CAD build for the part. Positions are in the model's coordinates, mm. A direction names the side the tool comes from. Give positions to 0.01 mm unless a question says otherwise; leave off trailing zeros. Write each loop counter-clockwise with the first axis right and the second up, starting at its lowest first coordinate (ties: lowest second). Pieces come first, ordered by that corner, then holes. Notation, with made-up numbers: (42.25, 40) - (63.25, 40) arc R21 cw to (63.25, 60) - close; hole circle Ø5 at (60.25, -23). An arc over 180 degrees is marked (long way). Answer as a JSON object with one key per item and string values.
from build123d import *

# Parameters (mm, degrees)
SKETCH1_R           = 0.19
SKETCH1_R_2         = 0.815
BOSS_EXTRUDE1_DEPTH = 1
SKETCH2_R           = 0.375
CUT_EXTRUDE1_DEPTH  = 0.75
SKETCH3_W           = 1.01
SKETCH3_H           = 1.01
CUT_EXTRUDE2_DEPTH  = 15
SKETCH4_R           = 0.125
CUT_EXTRUDE3_DEPTH  = 1.01
CHAMFER1_SIZE       = 0.05


with BuildPart() as part:
    # Sketch1 → Boss-Extrude1 (new body, symmetric)
    with BuildSketch(Plane.XY):
        with BuildLine():
            Line((0, 0), (0, 8))
            ThreePointArc((0, 8), (1.757359313, 12.242640687), (6, 14))
            Line((6, 14), (11.25, 14))
            Line((11.25, 14), (11.25, 10))
            Line((11.25, 10), (8, 10))
            ThreePointArc((8, 10), (5.171572875, 8.828427125), (4, 6))
            Line((4, 6), (4, 0))
            Line((4, 0), (0, 0))
        make_face()
        with Locations((0.5, 0.35)):
            Circle(SKETCH1_R, mode=Mode.SUBTRACT)
        with Locations((0.5, 1.15)):
            Circle(SKETCH1_R, mode=Mode.SUBTRACT)
        with Locations((9.56, 12)):
            Circle(SKETCH1_R_2, mode=Mode.SUBTRACT)
    extrude(amount=BOSS_EXTRUDE1_DEPTH, both=True)

    # Sketch2 → Cut-Extrude1 (cut)
    with BuildSketch(Plane(origin=(4, 0, 0), x_dir=(0, 0, -1), z_dir=(1, 0, 0))):
        with Locations((0, 0.75)):
            Circle(SKETCH2_R)
    extrude(amount=-CUT_EXTRUDE1_DEPTH, mode=Mode.SUBTRACT)

    # Sketch3 → Cut-Extrude2 (cut, through all)
    with BuildSketch(Plane(origin=(0, 14, 0), x_dir=(1, 0, 0), z_dir=(0, 1, 0))):
        with Locations((10.745, 0)):
            Rectangle(SKETCH3_W, SKETCH3_H)
    extrude(amount=-CUT_EXTRUDE2_DEPTH, mode=Mode.SUBTRACT)

    # Sketch4 → Cut-Extrude3 (cut)
    with BuildSketch(Plane(origin=(11.25, 0, 0), x_dir=(0, 0, -1), z_dir=(1, 0, 0))):
        with Locations((0.75, 13.5)):
            Circle(SKETCH4_R)
        with Locations((0.75, 10.5)):
            Circle(SKETCH4_R)
        with Locations((-0.75, 10.5)):
            Circle(SKETCH4_R)
        with Locations((-0.75, 13.5)):
            Circle(SKETCH4_R)
    extrude(amount=-CUT_EXTRUDE3_DEPTH, mode=Mode.SUBTRACT)

    # Chamfer1
    chamfer1_edges = [part.edges().sort_by_distance(p)[0] for p in [
        (9.625, 10, -1),
        (5.171572875, 8.828427125, -1),
        (4, 3, -1),
        (2, 0, -1),
        (5.171572875, 8.828427125, 1),
        (9.625, 10, 1),
        (11.25, 12, 1),
        (0.31, 0.35, -1),
        (0.31, 0.35, 1),
        (8.625, 14, 1),
        (0.31, 1.15, -1),
        (0.31, 1.15, 1),
        (1.757359313, 12.242640687, 1),
        (8.745, 12, -1),
        (8.745, 12, 1),
        (0, 4, 1),
        (2, 0, 1),
        (0, 4, -1),
        (4, 3, 1),
        (1.757359313, 12.242640687, -1),
        (8.625, 14, -1),
        (11.25, 12, -1),
    ]]
    chamfer(chamfer1_edges, length=CHAMFER1_SIZE)


solid = part.part
(1) Saw through at B-B, the plane x = 8.5. Give the cut face in (y, z).
Answer key:
{"outline": "(10, -0.95) - (10.05, -1) - (13.95, -1) - (14, -0.95) - (14, 0.95) - (13.95, 1) - (10.05, 1) - (10, 0.95) - close"}
(2) Pull direction X, two halves, no side cores. Call faces 4 (the face through (10.24, 13, 0)), 5 (the face through (9, 14, 0)), 6 (the face through (8.746, 12.036, -0.013)): pulls with the +X half, pulls with the -X half, needs draft (parallel to the pull), parting line crosses it, or undercut.
Answer key:
{"face 4": "pulls with the +X half", "face 5": "needs draft", "face 6": "undercut"}
(3) Probe L1, parallel to Y at x = 10.95, z = 0.75 (3 decimals); L2, parallel to Y at x = 0.5, z = 0.3; L3, parallel to X at y = 2, z = 0.85. List the from-to ranges inside material, lowest first. Write a range as [from, to].
Answer key:
{"L1": "y = [10, 10.375], [10.625, 13.375], [13.625, 14]", "L2": "y = [0, 0.16], [0.54, 0.96], [1.34, 10.4]", "L3": "x = [0, 4]"}
(4) 3-axis set-ups, long thin cutter, end or side, ignore diameter. For faces 1 (the face through (1.711, 12.196, 0.013)), 2 (the face through (10.24, 11, 0)), 3 (the face through (9, 10, 0)): which of +Z, -Z, +X, -X, +Y, -Y reach the whole face in a straight line?
Answer key:
{"face 1": "+Z, -Z, -X, +Y", "face 2": "+X, +Y, -Y", "face 3": "+Z, -Z, +X, -Y"}
(5) Flat gauge pins, fed straight in: P1, Ø0.6, axis at y = 1, z = 0, coming from the +X side; P2, Ø0.8, axis at y = 13.5, z = 0, coming from the +X side. Where does each tip first touch, or does it go through?
Answer key:
{"P1": "stops at x = 4", "P2": "stops at x = 10.24"}
(6) Saw through at A-A, the plane z = 0. Give the cut face in (x, y) (3 decimals).
Answer key:
{"outline": "(0, 0) - (4, 0) - (4, 0.375) - (3.25, 0.375) - (3.25, 1.125) - (4, 1.125) - (4, 6) arc R4 cw to (8, 10) - (10.24, 10) - (10.24, 11.551) arc R0.815 cw (long way) to (10.24, 12.449) - (10.24, 14) - (6, 14) arc R6 ccw to (0, 8) - close; hole circle Ø0.38 at (0.5, 0.35); hole circle Ø0.38 at (0.5, 1.15)"}
